Autodesk Fusion 360 part; units mm, degrees
sketch "Sketch1" plane through (0, 0, 0) normal (1, 0, 0) x (0, 1, 0)
  circle A0 centre (0, 0) radius 1.5
  circle A1 centre (0, -12) radius 1.5
  circle A2 centre (0, 0) radius 4.5
  circle A3 centre (0, -12) radius 3.5
  line L0 (-4.4843, -0.375) -> (-3.4878, -12.2917)
  line L1 (4.4843, -0.375) -> (3.4878, -12.2917)
  dimension "d1" = 3
  dimension "d2" = 3
  dimension "d3" = 12
  dimension "d4" = 7
  dimension "d5" = 9
extrude "Extrude1" add sketch "Sketch1" along normal blind 3
CAD build for the part. Positions are in the model's coordinates, mm. Coordinates: 2 decimals unless noted, no trailing zeros. Order: outer loops, then holes, each group sorted by start corner. A loop starts at its lowest first (then second) coordinate and runs counter-clockwise, first axis right, second up. Notation, with made-up numbers: (-11.75, 61) -> (31.25, 61) arc R29 cw to (31.25, 81) -> close; hole circle Ø1 at (-8, -11.75). An arc over 180 degrees is marked (long way). Use one line per item in the form item = value. Start each with the question number.
1) Drill centre lines: L1, parallel to Z at x = 2.15, y = 0; L2, parallel to Z at x = 0.55, y = -0.5; L3, parallel to Y at x = 1.6, z = -0.25. Where is each one in solid material? Low to high. Write a range as [from, to].
2) Band-saw the part on D-D on y = 1. Give the cut face in (x, z), then the cut area to 3 significant figures.
3) Band-saw the part on A-A on z = 0. Give the cut face in (x, y), then the cut area to 3 significant figures.
4) Drop flat-ended pins along their axis: pin 1 (2 mm diameter, centred on y = -1.5, z = -11.5, fed in from -X); pin 2 (1.5 mm diameter, centred on x = 0.5, z = -10, fed in from +Y); pin 3 (1 mm diameter, centred on x = 1.5, y = -2, fed in from +Z); pin 4 (1.5 mm diameter, centred on x = 0.5, z = 1.5, fed in from +Y). Give the stop position or say it passes through.
5) Band-saw the part on C-C on x = 2.3. Give the cut face in (y, z) (3 decimals), then the cut area to 3 significant figures.
6) Pull direction Z, two halves, no side cores. Call faces 1 (the cylindrical face through (1.5, 0.1, -15.5)), 2 (the flat face through (0, 0, -5)), 3 (the cylindrical face through (1.48, -1.5, -0.07)): +Z half, -Z half, draft (parallel to the pull), parting line (faces both ways), or undercut.
7) Band-saw the part on B-B on y = 0. Give the cut face in (x, z), then the cut area to 3 significant figures.
Entries:
q1.L1 = [-15.5, -13.5], [-10.5, -1.5], [1.5, 4.5]
q1.L2 = [-15.46, -13.41], [-10.59, -1.41], [1.41, 4.47]
q1.L3 = [-4.49, -1.48], [1.48, 4.49]
q2.outline = (0, -15.35) -> (3, -15.35) -> (3, -13.12) -> (0, -13.12) -> close; (0, -10.88) -> (3, -10.88) -> (3, -1.12) -> (0, -1.12) -> close; (0, 1.12) -> (3, 1.12) -> (3, 4.39) -> (0, 4.39) -> close
q2.area = 45.8 mm2
q3.outline = (0, -4.5) -> (3, -4.5) -> (3, -1.5) -> (0, -1.5) -> close; (0, 1.5) -> (3, 1.5) -> (3, 4.5) -> (0, 4.5) -> close
q3.area = 18.0 mm2
q4.pin_1 = 0
q4.pin_2 = 3.74
q4.pin_3 = 4.24
q4.pin_4 = 4.44
q5.outline = (-4.484, -0.375) -> (-3.488, -12.292) arc R3.5 ccw to (3.488, -12.292) -> (4.484, -0.375) arc R4.5 ccw (long way) to start; hole circle Ø3 at (0, -12); hole circle Ø3 at (0, 0)
q5.area = 133 mm2
q6.face_1 = -Z half
q6.face_2 = draft
q6.face_3 = undercut
q7.outline = (0, -15.5) -> (3, -15.5) -> (3, -13.5) -> (0, -13.5) -> close; (0, -10.5) -> (3, -10.5) -> (3, -1.5) -> (0, -1.5) -> close; (0, 1.5) -> (3, 1.5) -> (3, 4.5) -> (0, 4.5) -> close
q7.area = 42.0 mm2
